```python
from build123d import *

# Parameters (mm, degrees)
SKETCH1_W      = 8
SKETCH1_H      = 100
EXTRUDE1_DEPTH = 5
SKETCH2_R      = 1.55
EXTRUDE4_DEPTH = 5
SKETCH4_R      = 1.55
EXTRUDE6_DEPTH = 5
SKETCH5_W      = 4
SKETCH5_H      = 70
EXTRUDE7_DEPTH = 5
SKETCH6_W      = 1.530516358
SKETCH6_H      = 21.618543552
EXTRUDE8_DEPTH = 1


with BuildPart() as part:
    # Sketch1 → Extrude1 (new body)
    with BuildSketch(Plane(origin=(0, 0, 0), x_dir=(1, 0, 0), z_dir=(0, 1, 0))):
        Rectangle(SKETCH1_W, SKETCH1_H)
    extrude(amount=EXTRUDE1_DEPTH)

    # Sketch2 → Extrude4 (cut)
    with BuildSketch(Plane(origin=(0, 5, 0), x_dir=(1, 0, 0), z_dir=(0, 1, 0))):
        with Locations(Location((0, -46, 0), (0, 0, 270))):
            Circle(SKETCH2_R)
    extrude(amount=-EXTRUDE4_DEPTH, mode=Mode.SUBTRACT)

    # Sketch4 → Extrude6 (cut)
    with BuildSketch(Plane(origin=(0, 5, 0), x_dir=(1, 0, 0), z_dir=(0, 1, 0))):
        with Locations((0, -43.46)):
            Circle(SKETCH4_R)
        with Locations((0, -46)):
            Circle(SKETCH4_R)
        with Locations((0, 43)):
            Circle(SKETCH4_R)
        with Locations((0, 45.54)):
            Circle(SKETCH4_R)
    extrude(amount=-EXTRUDE6_DEPTH, mode=Mode.SUBTRACT)

    # Sketch5 → Extrude7 (cut)
    with BuildSketch(Plane(origin=(0, 5, 0), x_dir=(1, 0, 0), z_dir=(0, 1, 0))):
        with Locations((-2, 0)):
            Rectangle(SKETCH5_W, SKETCH5_H)
    extrude(amount=-EXTRUDE7_DEPTH, mode=Mode.SUBTRACT)

    # Sketch6 → Extrude8 (cut)
    with BuildSketch(Plane(origin=(0, 5, 0), x_dir=(1, 0, 0), z_dir=(0, 1, 0))):
        with Locations((2.112618746, 5.201364346)):
            Rectangle(SKETCH6_W, SKETCH6_H)
    extrude(amount=-EXTRUDE8_DEPTH, mode=Mode.SUBTRACT)


solid = part.part
```
The model under review builds one solid part; all positions refer to its coordinate system, in mm. A direction names the side the tool comes from. Round coordinates to 2 decimals unless told otherwise and drop trailing zeros. Loops run counter-clockwise (first coordinate to the right, second up) from the corner with the lowest first, then second, coordinate; pieces in that order, holes last. Notation, with made-up numbers: (61.5, 48.5) -> (66.5, 48.5) arc R14 ccw to (66.5, 60.5) -> close; hole circle Ø4 at (69.5, 12.5). An arc over 180 degrees is marked (long way). Answer in a Markdown table with one row per item.
1) Draft analysis for pull direction Z (two halves, no side actions). For faces 1 (the flat face through (-4, 2, 43)), 2 (the flat face through (0, 2, -50)), 3 (the flat face through (2, 4, -5)), 4 (the flat face through (0, 2, 50)), state which applies: pulls with the +Z half, pulls with the -Z half, needs draft (parallel to the pull), parting line crosses it, or undercut.
Taken from the geometry:
| item | result |
|---|---|
| face 1 | needs draft |
| face 2 | pulls with the -Z half |
| face 3 | undercut |
| face 4 | pulls with the +Z half |
2) For pin 1 Ø4 at (x, z) = (1.5, -7) entering from +Y; pin 2 Ø0.8 at (y, z) = (4.5, -10) entering from -X, all flat-tipped, find the tip position at first contact; note any pin that passes through.
Taken from the geometry:
| item | result |
|---|---|
| pin 1 | stops at y = 5 |
| pin 2 | stops at x = 0 |
3) Wall thickness on line 1 along Z through (x, y) = (2, 4.55); line 2 along X through (y, z) = (3.85, -45.54); line 3 along Z through (x, y) = (-1, 1.3): over which ranges is each line inside the solid? List them lowest first.
Taken from the geometry:
| item | result |
|---|---|
| line 1 | z = -50 to -16.01, 5.61 to 50 |
| line 2 | x = -4 to -1.55, 1.55 to 4 |
| line 3 | z = -50 to -46.72, -44.36 to -44.18, -41.82 to -35, 35 to 42.28, 44.64 to 44.82, 47.18 to 50 |
4) Consider section A-A, the plane x = -3. Write out the cut boundary in (y, z), plus the area to 3 significant figures.
Taken from the geometry:
| item | result |
|---|---|
| outline | (0, -50) -> (5, -50) -> (5, -35) -> (0, -35) -> close; (0, 35) -> (5, 35) -> (5, 50) -> (0, 50) -> close |
| area | 150 mm² |
5) Consider section C-C, the plane y = 1.5. Write out the cut boundary in (x, z).
Taken from the geometry:
| item | result |
|---|---|
| outline | (-4, -50) -> (4, -50) -> (4, 50) -> (-4, 50) -> (-4, 35) -> (0, 35) -> (0, -35) -> (-4, -35) -> close; hole (-0.89, -44.27) arc R1.55 ccw (long way) to (0.89, -44.27) arc R1.55 ccw (long way) to start; hole (-0.89, 44.73) arc R1.55 ccw (long way) to (0.89, 44.73) arc R1.55 ccw (long way) to start |
6) Consider section B-B, the plane z = 43.46. Write out the cut boundary in (x, y), plus the area to 3 significant figures.
Taken from the geometry:
| item | result |
|---|---|
| outline | (-4, 0) -> (-1.55, 0) -> (-1.55, 5) -> (-4, 5) -> close; (1.55, 0) -> (4, 0) -> (4, 5) -> (1.55, 5) -> close |
| area | 24.5 mm² |
7) Consider section D-D, the plane z = 10. Write out the cut boundary in (x, y).
Taken from the geometry:
| item | result |
|---|---|
| outline | (0, 0) -> (4, 0) -> (4, 5) -> (0, 5) -> close |
8) Tool access review of faces 5 (the flat face through (-2, 3, 35)), 6 (the flat face through (1, 5, -1)): name each direction out of +Z, -Z, +X, -X, +Y, -Y from which nothing blocks a thin tool from reaching the whole face with its end or side.
Taken from the geometry:
| item | result |
|---|---|
| face 5 | -X, +Y, -Y |
| face 6 | +Z, -Z, +X, -X, +Y |
